Check sheet for the drawn part. Datum: minimum x, y, z corner. Units: mm. Give positions to 0.01 mm unless a question says otherwise; leave off trailing zeros. Write each loop counter-clockwise with the first axis right and the second up, starting at its lowest first coordinate (ties: lowest second). Pieces come first, ordered by that corner, then holes. Notation, with made-up numbers: (75, 60.25) - (98, 60.25) arc R10 cw to (98, 77.25) - close; hole circle Ø10 at (74.5, 73). An arc over 180 degrees is marked (long way). Answer as a JSON object with one key per item and string values. Group by question number.
Item 1: Sectioned sample at A-A, the plane x = 34.5. Record the boundary of the cut face in (y, z).
Item 2: Scan lines: line 1 along X through (y, z) = (2, 23.5); line 2 along Z through (x, y) = (50, 1.65); line 3 along Y through (x, z) = (77, 23). Record each from-to range of solid material in increasing order. Write a range as [from, to].
Item 3: Go/stop test with flat-tipped pins: pin 1 (1.2 mm diameter, centred on x = 50, y = 2.5, fed in from +Z); pin 2 (1.2 mm diameter, centred on x = 47.5, y = 2.5, fed in from -Z); pin 3 (5 mm diameter, centred on x = 42, z = 18, fed in from +Y). Record where each tip stops, or that it passes through.
Item 4: Sectioned sample at B-B, the plane z = 10.5. Record the boundary of the cut face in (x, y), and give its area (3 significant figures).
Item 5: Draft check along Z on the marked faces 1 and 2. Enter one of: +Z half, -Z half, draft (parallel to the pull), parting line (faces both ways), or undercut.
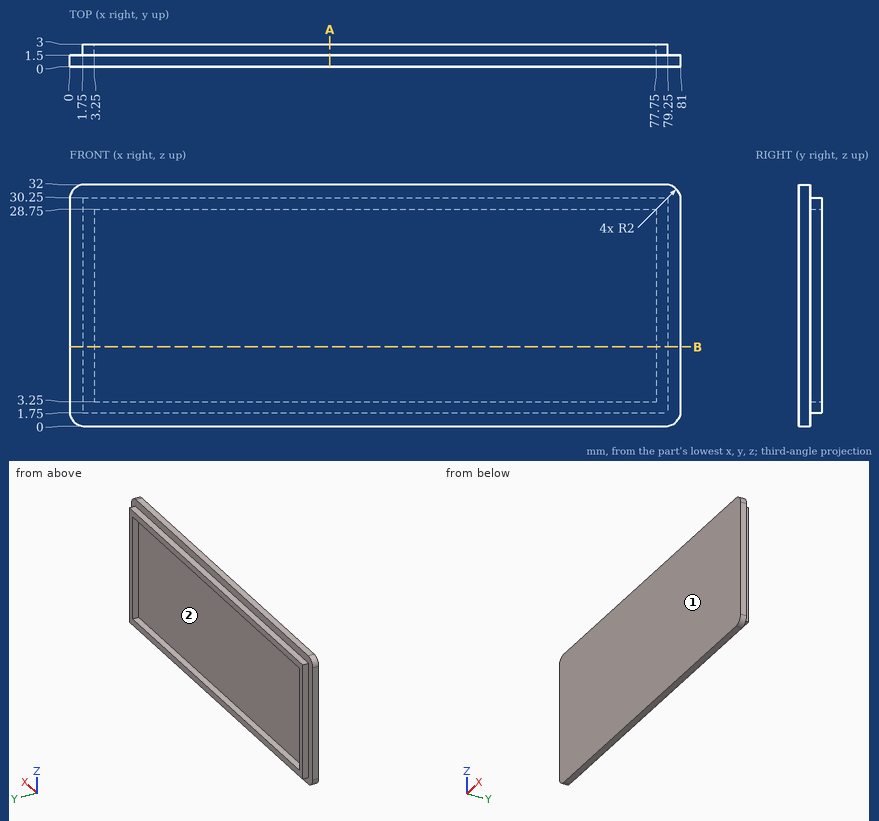
Geometry check:
{
 "1": {"outline": "(0, 0) - (1.5, 0) - (1.5, 1.75) - (3, 1.75) - (3, 3.25) - (1.5, 3.25) - (1.5, 28.75) - (3, 28.75) - (3, 30.25) - (1.5, 30.25) - (1.5, 32) - (0, 32) - close"},
 "2": {"line 1": "[1.75, 3.25], [77.75, 79.25]", "line 2": "[1.75, 3.25], [28.75, 30.25]", "line 3": "[0, 1.5]"},
 "3": {"pin 1": "z = 30.25", "pin 2": "z = 1.75", "pin 3": "y = 1.5"},
 "4": {"outline": "(0, 0) - (81, 0) - (81, 1.5) - (79.25, 1.5) - (79.25, 3) - (77.75, 3) - (77.75, 1.5) - (3.25, 1.5) - (3.25, 3) - (1.75, 3) - (1.75, 1.5) - (0, 1.5) - close", "area": "126 mm^2"},
 "5": {"face 1": "draft", "face 2": "undercut"}
}
